Work out the finished part from the listing and answer in its coordinate system (mm). A direction names the side the tool comes from. Round coordinates to 2 decimals unless told otherwise and drop trailing zeros. Write each loop counter-clockwise with the first axis right and the second up, starting at its lowest first coordinate (ties: lowest second). Pieces come first, ordered by that corner, then holes. Notation, with made-up numbers: M 78,42.25 L 119,42.25 A23 cw 119,77.25 Z; hole C -19,0 d7. An arc over 180 degrees is marked long. One line per item, written item: value. Start each with the question number.
Q1. Given pin 1 Ø4 at (x, z) = (-37.5, -15.5) entering from +Y; pin 2 Ø2 at (x, z) = (-27.5, 13) entering from +Y; pin 3 Ø1.5 at (x, y) = (13.5, 5) entering from -Z; pin 4 Ø2.5 at (y, z) = (4.5, -0.5) entering from -X, each flat-ended and moving along its own axis, determine where each tip first touches the part or whether it passes through.
Q2. Find section B-B (x = 21). Write down the section's boundary in (y, z).
Q3. Find section A-A (z = -15.5). Write down the section's boundary in (x, y).
Q4. A tool of negligible diameter and unlimited length cuts with its end or side. For faces 4 (the flat face through (-1, 4, -12.1)), 5 (the flat face through (36.85, 4, 0)), 6 (the flat face through (1, 4, 12.7)), 7 (the flat face through (0, 6.5, 0)), 8 (the flat face through (-36.85, 4, 0)), from which of +Z, -Z, +X, -X, +Y, -Y can it reach the whole face along a straight path? Write none if from no direction.
Q5. Find section C-C (z = -4.5). Write down the section's boundary in (x, y).
Q6. Find section D-D (y = 4.75). Write down the section's boundary in (x, z).
Q7. The mould has two halves that part along Z. Classify faces 1 (the cylindrical face through (-36.28, 0.79, 15.23)), 2 (the flat face through (-1, 1, -18)), 3 (the flat face through (-3, 1.6, -13)): released by +Z, released by -Z, zero draft, split by the parting line, or undercut.
Q8. Consider probe 1 along Z at (x, y) = (37.5, 0.75); probe 2 along X at (y, z) = (0.65, -15.5); probe 3 along Y at (x, z) = (10.5, 13.5). Determine where each line is inside the solid, lowest interval first.
Autodesk Inventor part; units mm, degrees
ref_plane "YZ Plane" through (0, 0, 0) normal (1, 0, 0) x (0, 1, 0)
ref_plane "XZ Plane" through (0, 0, 0) normal (0, 1, 0) x (-1, 0, 0)
ref_plane "XY Plane" through (0, 0, 0) normal (0, 0, 1) x (1, 0, 0)
sketch "Sketch1" plane through (0, 0, 0) normal (0, 1, 0) x (-1, 0, 0)
  line L0 (-40, 18) -> (40, 18)
  line L1 (40, 18) -> (40, -18)
  line L2 (40, -18) -> (-40, -18)
  line L3 (-40, -18) -> (-40, 18)
  line L4 (-40, 18) -> (40, -18) construction
  line L5 (40, 18) -> (-40, -18) construction
  point P0 (0, 0)
  dimension "d0" = 80
  dimension "d1" = 36
extrude "Extrusion1" add sketch "Sketch1" along normal blind 1.6
sketch "Sketch2" plane through (0, 1.6, 0) normal (0, 1, 0) x (1, 0, 0)
  line L0 (-40, -18) -> (40, -18) construction
  line L1 (40, -18) -> (40, 18) construction
  line L2 (40, 18) -> (-40, 18) construction
  line L3 (-40, 18) -> (-40, -18) construction
  point P0 (0, 0)
  point P1 (-37.5, 15.5)
  point P2 (37.5, 15.5)
  point P3 (-37.5, -15.5)
  point P4 (37.5, -15.5)
  dimension "d4" = 75
  dimension "d5" = 31
  dimension "d6" = 2.5
  dimension "d7" = 2.5
hole "Hole1" at (-37.5, 1.6, -15.5) at (37.5, 1.6, -15.5) at (-37.5, 1.6, 15.5) at (37.5, 1.6, 15.5) direction (0, -1, 0) diameter 2.5 end through all
sketch "Sketch3" plane through (0, 1.6, 0) normal (0, 1, 0) x (1, 0, 0)
  line L0 (36.85, -12.7) -> (-36.85, -12.7)
  line L1 (-36.85, -12.7) -> (-36.85, 12.1)
  line L2 (-36.85, 12.1) -> (36.85, 12.1)
  line L3 (36.85, 12.1) -> (36.85, -12.7)
  line L4 (36.85, -12.7) -> (-36.85, 12.1) construction
  line L5 (-36.85, -12.7) -> (36.85, 12.1) construction
  circle A0 centre (-37.5, -15.5) radius 1.25 construction
  circle A1 centre (-37.5, 15.5) radius 1.25 construction
  circle A2 centre (37.5, 15.5) radius 1.25 construction
  circle A3 centre (37.5, -15.5) radius 1.25 construction
  line L6 (-40, -18) -> (40, -18) construction
  line L7 (40, -18) -> (40, 18) construction
  line L8 (40, 18) -> (-40, 18) construction
  line L9 (-40, 18) -> (-40, -18) construction
  point P0 (0, 0)
  point P1 (0, -0.3)
  dimension "d15" = 73.7
  dimension "d16" = 24.8
  dimension "d17" = 5.9
  dimension "d18" = 3.15
extrude "Extrusion2" add sketch "Sketch3" along normal blind 5
sketch "Sketch4" plane through (0, 6.6, 0) normal (0, 1, 0) x (1, 0, 0)
  line L0 (32.25, -7.7) -> (-32.25, -7.7)
  line L1 (-32.25, -7.7) -> (-32.25, 7.1)
  line L2 (-32.25, 7.1) -> (32.25, 7.1)
  line L3 (32.25, 7.1) -> (32.25, -7.7)
  line L4 (32.25, -7.7) -> (-32.25, 7.1) construction
  line L5 (-32.25, -7.7) -> (32.25, 7.1) construction
  line L6 (-36.85, -12.7) -> (-36.85, 12.1) construction
  line L7 (-36.85, 12.1) -> (36.85, 12.1) construction
  line L8 (36.85, 12.1) -> (36.85, -12.7) construction
  line L9 (36.85, -12.7) -> (-36.85, -12.7) construction
  circle A0 centre (-37.5, -15.5) radius 1.25 construction
  circle A1 centre (-37.5, 15.5) radius 1.25 construction
  circle A2 centre (37.5, 15.5) radius 1.25 construction
  circle A3 centre (37.5, -15.5) radius 1.25 construction
  line L10 (-40, -18) -> (40, -18) construction
  line L11 (40, -18) -> (40, 18) construction
  line L12 (40, 18) -> (-40, 18) construction
  line L13 (-40, 18) -> (-40, -18) construction
  point P0 (0, 0)
  point P1 (0, -0.3)
  dimension "d21" = 64.5
  dimension "d22" = 14.8
  dimension "d23" = 10.9
  dimension "d24" = 7.75
extrude "Extrusion3" cut sketch "Sketch4" against normal blind 0.1
sketch "Sketch5" plane through (0, 6.5, 0) normal (0, 1, 0) x (1, 0, 0)
  line L0 (-28.1, 5.45) -> (28.1, 5.45) construction
  line L1 (28.1, 5.45) -> (28.1, -6.05) construction
  line L2 (28.1, -6.05) -> (-28.1, -6.05) construction
  line L3 (-28.1, -6.05) -> (-28.1, 5.45) construction
  line L4 (32.25, -7.7) -> (-32.25, -7.7) construction
  line L5 (32.25, 7.1) -> (32.25, -7.7) construction
  line L6 (-32.25, 7.1) -> (32.25, 7.1) construction
  line L7 (-32.25, -7.7) -> (-32.25, 7.1) construction
  line L8 (-36.85, -12.7) -> (-36.85, 12.1) construction
  line L9 (-36.85, 12.1) -> (36.85, 12.1) construction
  line L10 (36.85, 12.1) -> (36.85, -12.7) construction
  line L11 (36.85, -12.7) -> (-36.85, -12.7) construction
  circle A0 centre (-37.5, -15.5) radius 1.25 construction
  circle A1 centre (-37.5, 15.5) radius 1.25 construction
  circle A2 centre (37.5, 15.5) radius 1.25 construction
  circle A3 centre (37.5, -15.5) radius 1.25 construction
  line L12 (-40, -18) -> (40, -18) construction
  line L13 (40, -18) -> (40, 18) construction
  line L14 (40, 18) -> (-40, 18) construction
  line L15 (-40, 18) -> (-40, -18) construction
  line L16 (32.25, 7.1) -> (32.25, -7.7) construction
  line L17 (32.25, -7.7) -> (-32.25, -7.7) construction
  line L18 (-32.25, -7.7) -> (-32.25, 7.1) construction
  line L19 (-32.25, 7.1) -> (32.25, 7.1) construction
  line L20 (-36.85, -12.7) -> (36.85, -12.7) construction
  line L21 (36.85, -12.7) -> (36.85, 12.1) construction
  line L22 (36.85, 12.1) -> (-36.85, 12.1) construction
  line L23 (-36.85, 12.1) -> (-36.85, -12.7) construction
  point P0 (0, 0)
  dimension "d27" = 56.2
  dimension "d28" = 11.5
  dimension "d29" = 12.55
  dimension "d30" = 11.9
properties part number "LCD Display"
The answers:
1. pin 1: y = 1.6
1. pin 2: y = 6.6
1. pin 3: z = -12.1
1. pin 4: x = -36.85
2. outline: M 0,-18 L 1.6,-18 L 1.6,-12.1 L 6.6,-12.1 L 6.6,-7.1 L 6.5,-7.1 L 6.5,7.7 L 6.6,7.7 L 6.6,12.7 L 1.6,12.7 L 1.6,18 L 0,18 Z
3. outline: M -40,0 L -38.75,0 L -38.75,1.6 L -40,1.6 Z; M -36.25,0 L 36.25,0 L 36.25,1.6 L -36.25,1.6 Z; M 38.75,0 L 40,0 L 40,1.6 L 38.75,1.6 Z
4. face 4: -Z, +X, -X, +Y
4. face 5: +Z, -Z, +X, +Y
4. face 6: +Z, +X, -X, +Y
4. face 7: +Y
4. face 8: +Z, -Z, -X, +Y
5. outline: M -40,0 L 40,0 L 40,1.6 L 36.85,1.6 L 36.85,6.6 L 32.25,6.6 L 32.25,6.5 L -32.25,6.5 L -32.25,6.6 L -36.85,6.6 L -36.85,1.6 L -40,1.6 Z
6. outline: M -36.85,-12.1 L 36.85,-12.1 L 36.85,12.7 L -36.85,12.7 Z
7. face 1: undercut
7. face 2: released by -Z
7. face 3: zero draft
8. probe 1: -18 to -16.75, -14.25 to 14.25, 16.75 to 18
8. probe 2: -40 to -38.75, -36.25 to 36.25, 38.75 to 40
8. probe 3: 0 to 1.6
